```python
from build123d import *

# Parameters (mm, degrees)
SKETCH1_W           = 148
SKETCH1_H           = 87
BOSS_EXTRUDE1_DEPTH = 20
SHELL1_T            = -5
BOSS_EXTRUDE2_REACH = 157.551
SKETCH2_W           = 3
SKETCH2_H           = 77
SKETCH3_W           = 25
SKETCH3_H           = 5
CUT_EXTRUDE1_DEPTH  = 8


with BuildPart() as part:
    # Sketch1 → Boss-Extrude1 (new body)
    with BuildSketch(Plane(origin=(0, 0, 0), x_dir=(1, 0, 0), z_dir=(0, 1, 0))):
        with Locations((74, 0)):
            Rectangle(SKETCH1_W, SKETCH1_H)
    extrude(amount=BOSS_EXTRUDE1_DEPTH)

    # Shell1
    shell1_openings = [part.faces().sort_by_distance(p)[0] for p in [
        (74, 20, 0),
    ]]
    offset(amount=SHELL1_T, openings=shell1_openings, kind=Kind.INTERSECTION)

    # Sketch2 → Boss-Extrude2 (add, up to next)
    with BuildSketch(Plane(origin=(0, 20, 0), x_dir=(1, 0, 0), z_dir=(0, 1, 0)), mode=Mode.PRIVATE) as boss_extrude2_sk1:
        with Locations((50.5, 0)):
            Rectangle(SKETCH2_W, SKETCH2_H)
    boss_extrude2_tool1 = extrude(boss_extrude2_sk1.sketch, amount=-BOSS_EXTRUDE2_REACH, mode=Mode.PRIVATE) - part.part
    # Sketch2 → Boss-Extrude2 (add, up to next)
    with BuildSketch(Plane(origin=(0, 20, 0), x_dir=(1, 0, 0), z_dir=(0, 1, 0)), mode=Mode.PRIVATE) as boss_extrude2_sk2:
        with Locations((97.5, 0)):
            Rectangle(SKETCH2_W, SKETCH2_H)
    boss_extrude2_tool2 = extrude(boss_extrude2_sk2.sketch, amount=-BOSS_EXTRUDE2_REACH, mode=Mode.PRIVATE) - part.part
    add(boss_extrude2_tool1.solids().sort_by_distance((50.5, 20, 0))[0])
    add(boss_extrude2_tool2.solids().sort_by_distance((97.5, 20, 0))[0])

    # Sketch3 → Cut-Extrude1 (cut)
    with BuildSketch(Plane(origin=(0, 20, 0), x_dir=(1, 0, 0), z_dir=(0, 1, 0))):
        with Locations((25.5, 41)):
            Rectangle(SKETCH3_W, SKETCH3_H)
        with Locations((72.5, 41)):
            Rectangle(SKETCH3_W, SKETCH3_H)
        with Locations((119.5, 41)):
            Rectangle(SKETCH3_W, SKETCH3_H)
    extrude(amount=-CUT_EXTRUDE1_DEPTH, mode=Mode.SUBTRACT)


solid = part.part
```
Work out the finished part from the listing and answer in its coordinate system (mm). A direction names the side the tool comes from. Coordinates: 2 decimals unless noted, no trailing zeros. Write each loop counter-clockwise with the first axis right and the second up, starting at its lowest first coordinate (ties: lowest second). Pieces come first, ordered by that corner, then holes.
Q1. Which of the six approach directions +Z, -Z, +X, -X, +Y, -Y give full straight-line access (tool end or side, diameter ignored) to faces 1 (the face through (72, 12, -41)), 2 (the face through (96, 13, 1)), 3 (the face through (148, 10, 1))?
Q2. A cutting plane is placed at B-B, the plane y = 9.5. Give the vertices of the cut face in (x, z), then the cut area to 3 significant figures.
Q3. Each of these flat-tipped pins is pushed along its axis until it touches: pin 1 Ø13 at (x, z) = (124, 6) entering from +Y; pin 2 Ø10 at (x, z) = (118.5, -25.5) entering from -Y; pin 3 Ø2 at (x, y) = (114, 15) entering from -Z; pin 4 Ø2.5 at (x, z) = (26.5, -41) entering from +Y. Where does it stop, or does it pass through?
Q4. A cutting plane is placed at C-C, the plane z = 23. Give the vertices of the cut face in (x, y).
Q5. Find the intervals of material crossed by line 1 (X direction, y = 17, z = -36); line 2 (Z direction, x = 42, y = 13); line 3 (Y direction, x = 113, z = 17.5), in increasing order.
Q6. A cutting plane is placed at A-A, the plane x = 36.5. Give the vertices of the cut face in (y, z).
Findings below:
1. face 1: -Z, +Y
1. face 2: +Y
1. face 3: +Z, -Z, +X, +Y, -Y
2. outline: (0, -43.5) - (148, -43.5) - (148, 43.5) - (0, 43.5) - close; hole (5, -38.5) - (49, -38.5) - (49, 38.5) - (5, 38.5) - close; hole (52, -38.5) - (96, -38.5) - (96, 38.5) - (52, 38.5) - close; hole (99, -38.5) - (143, -38.5) - (143, 38.5) - (99, 38.5) - close
2. area: 2,710 mm2
3. pin 1: stops at y = 5
3. pin 2: stops at y = 0
3. pin 3: stops at z = 38.5
3. pin 4: stops at y = 12
4. outline: (0, 0) - (148, 0) - (148, 20) - (143, 20) - (143, 5) - (99, 5) - (99, 20) - (96, 20) - (96, 5) - (52, 5) - (52, 20) - (49, 20) - (49, 5) - (5, 5) - (5, 20) - (0, 20) - close
5. line 1: x = 0 to 5, 49 to 52, 96 to 99, 143 to 148
5. line 2: z = -43.5 to -38.5, 38.5 to 43.5
5. line 3: y = 0 to 5
6. outline: (0, -43.5) - (12, -43.5) - (12, -38.5) - (5, -38.5) - (5, 38.5) - (20, 38.5) - (20, 43.5) - (0, 43.5) - close
